```python
from build123d import *

# Parameters (mm, degrees)
BOSS_EXTRUDE1_DEPTH = 38.1
SKETCH2_R           = 6.35
CUT_EXTRUDE1_DEPTH  = 277.206752271
SKETCH3_R           = 9.525
CUT_EXTRUDE3_DEPTH  = 35.56
SKETCH5_R           = 6.35
BOSS_EXTRUDE2_DEPTH = 12.7
SKETCH6_R           = 6.35
CUT_EXTRUDE4_DEPTH  = 279.243059213


with BuildPart() as part:
    # Sketch1 → Boss-Extrude1 (new body)
    with BuildSketch(Plane.XY):
        with BuildLine():
            Line((0, 0), (0, 203.2))
            ThreePointArc((0, 203.2), (50.8, 254), (101.6, 203.2))
            Line((101.6, 203.2), (101.6, 0))
            ThreePointArc((101.6, 0), (50.8, -50.8), (0, 0))
        make_face()
    extrude(amount=BOSS_EXTRUDE1_DEPTH)

    # Sketch2 → Cut-Extrude1 (cut, through all)
    with BuildSketch(Plane.XY.offset(38.1)):
        with Locations((50.8, 203.2)):
            Circle(SKETCH2_R)
        with Locations((50.8, 0)):
            Circle(SKETCH2_R)
    extrude(amount=-CUT_EXTRUDE1_DEPTH, mode=Mode.SUBTRACT)

    # Sketch3 → Cut-Extrude3 (cut)
    with BuildSketch(Plane.XY.offset(38.1)):
        with Locations((50.327847378, 152.4)):
            Circle(SKETCH3_R)
        with Locations((50.327847378, 50.8)):
            Circle(SKETCH3_R)
    extrude(amount=-CUT_EXTRUDE3_DEPTH, mode=Mode.SUBTRACT)

    # Sketch5 → Boss-Extrude2 (add)
    with BuildSketch(Plane.XY.offset(38.1)):
        with Locations((50.327847378, 101.6)):
            Circle(SKETCH5_R)
    extrude(amount=BOSS_EXTRUDE2_DEPTH)

    # Sketch6 → Cut-Extrude4 (cut, through all)
    with BuildSketch(Plane(origin=(101.6, 0, 0), x_dir=(0, 0, -1), z_dir=(1, 0, 0))):
        with Locations((-19.05, 101.6)):
            Circle(SKETCH6_R)
    extrude(amount=-CUT_EXTRUDE4_DEPTH, mode=Mode.SUBTRACT)


solid = part.part
```
The model under review builds one solid part; all positions refer to its coordinate system, in mm. A direction names the side the tool comes from. Round coordinates to 2 decimals unless told otherwise and drop trailing zeros. Loops run counter-clockwise (first coordinate to the right, second up) from the corner with the lowest first, then second, coordinate; pieces in that order, holes last. Notation, with made-up numbers: (85.25, 78) - (90.25, 78) arc R21 ccw to (90.25, 108) - close; hole circle Ø11 at (16.25, 74.5). An arc over 180 degrees is marked (long way). Write each question's results on one line, items separated by ' | '. Start each with the question number.
Q1. Draft analysis for pull direction Y (two halves, no side actions). For faces 3 (the cylindrical face through (51.511, 107.896, 19.877)), 4 (the flat face through (50, 51, 2.54)), 5 (the cylindrical face through (53.742, 106.954, 44.361)), 6 (the flat face through (40, 104, 38.1)), state which applies: pulls with the +Y half, pulls with the -Y half, needs draft (parallel to the pull), parting line crosses it, or undercut.
Q2. Tool access review of faces 1 (the cylindrical face through (55.45, 58.83, 20.57)), 2 (the cylindrical face through (54.214, 208.554, 19.317)): name each direction out of +Z, -Z, +X, -X, +Y, -Y from which nothing blocks a thin tool from reaching the whole face with its end or side.
Q3. Take a section at C-C on x = 50.8. Give the boundary of the cut face in (y, z), plus the area to 3 significant figures.
Q4. Take a section at B-B on y = 101.6. Give the boundary of the cut face in (x, z), plus the area to 3 significant figures.
Q5. Take a section at D-D on y = 152.4. Give the boundary of the cut face in (x, z), plus the area to 3 significant figures.
Q6. Wall thickness on line 1 along Y through (x, z) = (50.8, 9.5); line 2 along Y through (x, z) = (50.8, 22.5); line 3 along Y through (x, z) = (50.8, 16): over which ranges is each line inside the solid? List them lowest first. Write a range as [from, to].
Q7. Take a section at A-A on z = 19.05. Give the boundary of the cut face in (x, y) (3 decimals), plus the area to 3 significant figures.
Q8. Insertion check: P1, Ø12, axis at y = 3.5, z = 5, coming from the -X side; P2, Ø9.5, axis at x = 51, y = 150.5, coming from the +Z side; P3, Ø4, axis at y = 178.5, z = 40.5, coming from the -X side; P4, Ø21, axis at x = 47.5, y = 55.5, coming from the +Z side. Each pin has a flat end and moves straight along its axis. Give the tip position at first contact, or say it passes through.
Data:
1) face 3: undercut | face 4: undercut | face 5: parting line crosses it | face 6: needs draft
2) face 1: +Z | face 2: +Z, -Z
3) outline: (-50.8, 0) - (-6.35, 0) - (-6.35, 38.1) - (-50.8, 38.1) - close; (6.35, 0) - (196.85, 0) - (196.85, 38.1) - (161.91, 38.1) - (161.91, 2.54) - (142.89, 2.54) - (142.89, 38.1) - (107.93, 38.1) - (107.93, 50.8) - (95.27, 50.8) - (95.27, 38.1) - (60.31, 38.1) - (60.31, 2.54) - (41.29, 2.54) - (41.29, 38.1) - (6.35, 38.1) - close; (209.55, 0) - (254, 0) - (254, 38.1) - (209.55, 38.1) - close; hole circle Ø12.7 at (101.6, 19.05) | area: 9,330 mm²
4) outline: (0, 0) - (101.6, 0) - (101.6, 12.7) - (0, 12.7) - close; (0, 25.4) - (101.6, 25.4) - (101.6, 38.1) - (56.68, 38.1) - (56.68, 50.8) - (43.98, 50.8) - (43.98, 38.1) - (0, 38.1) - close | area: 2,740 mm²
5) outline: (0, 0) - (101.6, 0) - (101.6, 38.1) - (59.85, 38.1) - (59.85, 2.54) - (40.8, 2.54) - (40.8, 38.1) - (0, 38.1) - close | area: 3,190 mm²
6) line 1: y = [-50.8, -6.35], [6.35, 41.29], [60.31, 142.89], [161.91, 196.85], [209.55, 254] | line 2: y = [-50.8, -6.35], [6.35, 41.29], [60.31, 96.27], [106.93, 142.89], [161.91, 196.85], [209.55, 254] | line 3: y = [-50.8, -6.35], [6.35, 41.29], [60.31, 96.03], [107.17, 142.89], [161.91, 196.85], [209.55, 254]
7) outline: (0, 0) arc R50.8 ccw to (101.6, 0) - (101.6, 95.25) - (0, 95.25) - close; (0, 107.95) - (101.6, 107.95) - (101.6, 203.2) arc R50.8 ccw to (0, 203.2) - close; hole circle Ø19.05 at (50.328, 50.8); hole circle Ø19.05 at (50.328, 152.4); hole circle Ø12.7 at (50.8, 0); hole circle Ø12.7 at (50.8, 203.2) | area: 26,600 mm²
8) P1: stops at x = 0 | P2: stops at z = 2.54 | P3: passes through | P4: stops at z = 38.1
